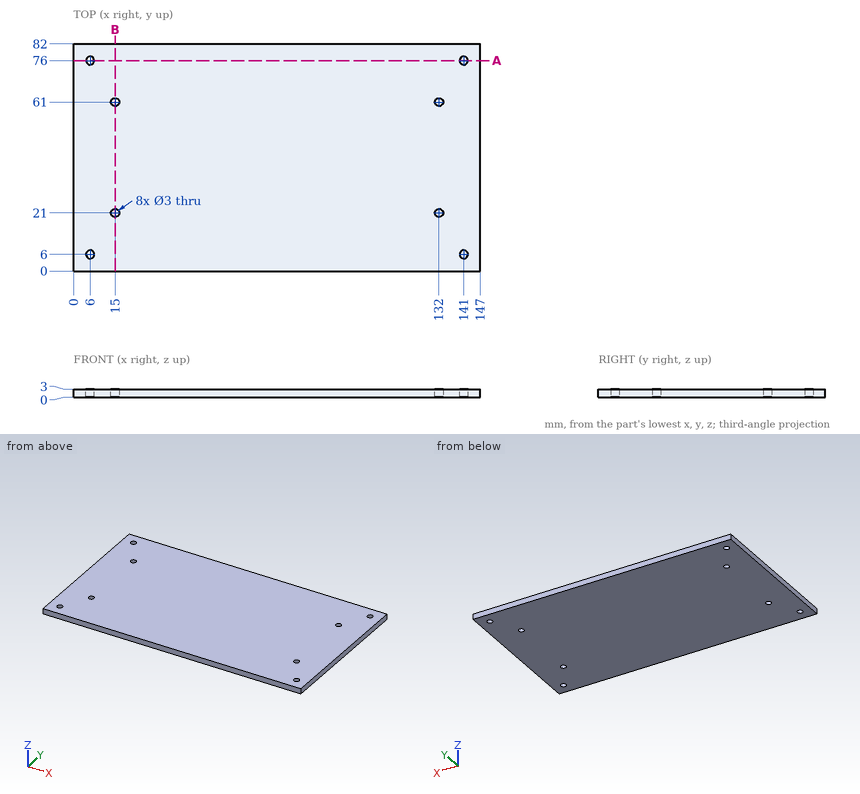
Job drawing, mm, ordinate dimensions from the low corner. One solid piece. Coordinates: 2 decimals unless noted, no trailing zeros. Write each loop counter-clockwise with the first axis right and the second up, starting at its lowest first coordinate (ties: lowest second). Pieces come first, ordered by that corner, then holes.
Item 1: Pin check, flat tips, straight feed: pin 1 (2.5 mm diameter, centred on x = 15, y = 21, fed in from +Z); pin 2 (3.5 mm diameter, centred on x = 141, y = 76, fed in from +Z). Stop position of each tip, or through.
Item 2: Probe line 1 (Y direction, x = 6, z = 0.9); line 2 (X direction, y = 76, z = 2.25); line 3 (Y direction, x = 15, z = 1.55). List the from-to ranges inside material, lowest first.
Item 3: Slice it at A-A (y = 76). Write the cut outline in (x, z).
Item 4: Slice it at B-B (x = 15). Write the cut outline in (y, z), and give its area (3 significant figures).
Results found:
1. pin 1: passes through
1. pin 2: stops at z = 3
2. line 1: y = 0 to 4.5, 7.5 to 74.5, 77.5 to 82
2. line 2: x = 0 to 4.5, 7.5 to 139.5, 142.5 to 147
2. line 3: y = 0 to 19.5, 22.5 to 59.5, 62.5 to 82
3. outline: (0, 0) - (4.5, 0) - (4.5, 3) - (0, 3) - close; (7.5, 0) - (139.5, 0) - (139.5, 3) - (7.5, 3) - close; (142.5, 0) - (147, 0) - (147, 3) - (142.5, 3) - close
4. outline: (0, 0) - (19.5, 0) - (19.5, 3) - (0, 3) - close; (22.5, 0) - (59.5, 0) - (59.5, 3) - (22.5, 3) - close; (62.5, 0) - (82, 0) - (82, 3) - (62.5, 3) - close
4. area: 228 mm2
